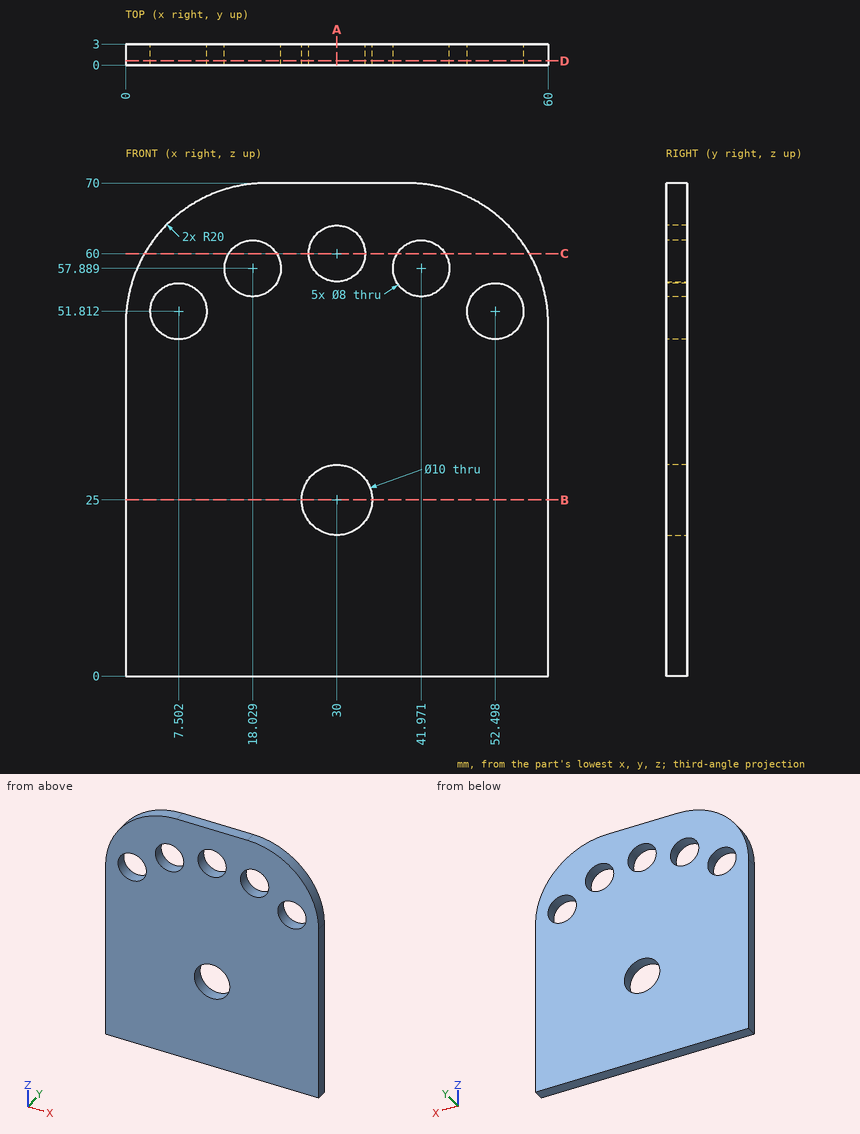
For this review, use the dimensioned drawing (mm, ordinates from the lowest corner) and the shaded views. Coordinates: 2 decimals unless noted, no trailing zeros. Write each loop counter-clockwise with the first axis right and the second up, starting at its lowest first coordinate (ties: lowest second). Pieces come first, ordered by that corner, then holes. Notation, with made-up numbers: (22, -22.5) - (27, -22.5) arc R28 cw to (27, 16.5) - close; hole circle Ø5 at (37.25, -2). An arc over 180 degrees is marked (long way). One line per item, written item: value.
1) To check wall thickness, follow probe 1 along X at (y, z) = (1.8, 22); probe 2 along X at (y, z) = (0.9, 53) (1 decimal); probe 3 along X at (y, z) = (2.4, 49.5) (1 decimal). State the ranges of each line that lie inside material, in increasing order.
Answer sheet:
probe 1: x = 0 to 26, 34 to 60
probe 2: x = 0.2 to 3.7, 11.3 to 48.7, 56.3 to 59.8
probe 3: x = 0 to 4.2, 10.8 to 49.2, 55.8 to 60
2) Add section C-C (z = 60). State the section outline as (x, y) points.
Answer sheet:
outline: (2.68, 0) - (14.63, 0) - (14.63, 3) - (2.68, 3) - close; (21.43, 0) - (26, 0) - (26, 3) - (21.43, 3) - close; (34, 0) - (38.57, 0) - (38.57, 3) - (34, 3) - close; (45.37, 0) - (57.32, 0) - (57.32, 3) - (45.37, 3) - close
3) Add section A-A (x = 30). State the section outline as (y, z) points, plus the area to 3 significant figures.
Answer sheet:
outline: (0, 0) - (3, 0) - (3, 20) - (0, 20) - close; (0, 30) - (3, 30) - (3, 56) - (0, 56) - close; (0, 64) - (3, 64) - (3, 70) - (0, 70) - close
area: 156 mm2
4) Add section B-B (z = 25). State the section outline as (x, y) points, plus the area to 3 significant figures.
Answer sheet:
outline: (0, 0) - (25, 0) - (25, 3) - (0, 3) - close; (35, 0) - (60, 0) - (60, 3) - (35, 3) - close
area: 150 mm2
5) Insertion check: pin 1 (7 mm diameter, centred on x = 30, z = 60, fed in from -Y); pin 2 (1 mm diameter, centred on y = 1, z = 52, fed in from +X). Each pin has a flat end and moves straight along its axis. Give the tip position at first contact, or say it passes through.
Answer sheet:
pin 1: passes through
pin 2: stops at x = 59.94
6) Add section D-D (y = 0.6). State the section outline as (x, z) points, plus the area to 3 significant figures.
Answer sheet:
outline: (0, 0) - (60, 0) - (60, 50) arc R20 ccw to (40, 70) - (20, 70) arc R20 ccw to (0, 50) - close; hole circle Ø8 at (7.5, 51.81); hole circle Ø8 at (18.03, 57.89); hole circle Ø10 at (30, 25); hole circle Ø8 at (30, 60); hole circle Ø8 at (41.97, 57.89); hole circle Ø8 at (52.5, 51.81)
area: 3,700 mm2
